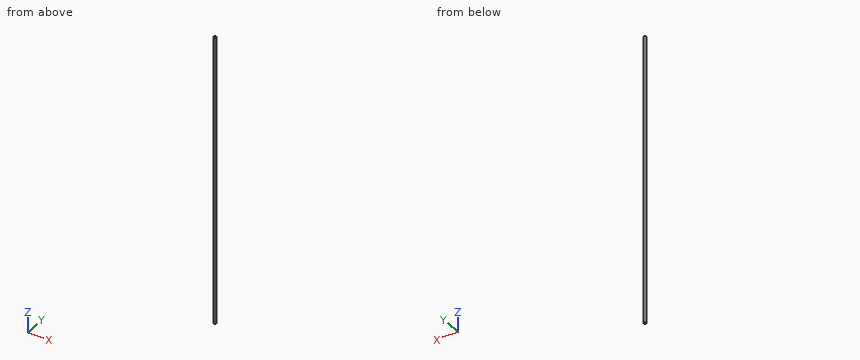
```python
from build123d import *

# Parameters (mm, degrees)
SKETCH1_R           = 0.975
BOSS_EXTRUDE1_DEPTH = 244.38
SKETCH2_W           = 1
SKETCH2_H           = 1
CUT_EXTRUDE1_DEPTH  = 5


with BuildPart() as part:
    # Sketch1 → Boss-Extrude1 (new body)
    with BuildSketch(Plane.XY):
        Circle(SKETCH1_R)
    extrude(amount=BOSS_EXTRUDE1_DEPTH)

    # Sketch2 → Cut-Extrude1 (cut)
    with BuildSketch(Plane.XY):
        Rectangle(SKETCH2_W, SKETCH2_H)
    extrude(amount=CUT_EXTRUDE1_DEPTH, mode=Mode.SUBTRACT)


solid = part.part
```
Geometry check sheet. Reference: the model listing, model coordinates, mm. Give positions to 0.01 mm unless a question says otherwise; leave off trailing zeros. Order: outer loops, then holes, each group sorted by start corner. A loop starts at its lowest first (then second) coordinate and runs counter-clockwise, first axis right, second up. Notation, with made-up numbers: (87, 61.25) -> (112, 61.25) arc R31 cw to (112, 90.25) -> close; hole circle Ø11 at (-8.75, 1.25). An arc over 180 degrees is marked (long way). Write each question's results on one line, items separated by ' | '. Start each with the question number.
(1) Scan lines: line 1 (Z direction, x = -0.2, y = 0.05); line 2 (Y direction, x = 0.3, z = 168); line 3 (Y direction, x = -0.2, z = 133). Record each from-to range of solid material in increasing order.
(2) Sectioned sample at B-B (z = 112). Enter the section's corners in (x, y) (3 decimals).
(3) Sectioned sample at A-A (x = -0.15). Enter the section's corners in (y, z).
Answer below:
1) line 1: 5 to 244.38 | line 2: -0.93 to 0.93 | line 3: -0.95 to 0.95
2) outline: circle Ø1.95 at (0, 0)
3) outline: (-0.96, 0) -> (-0.5, 0) -> (-0.5, 5) -> (0.5, 5) -> (0.5, 0) -> (0.96, 0) -> (0.96, 244.38) -> (-0.96, 244.38) -> close
